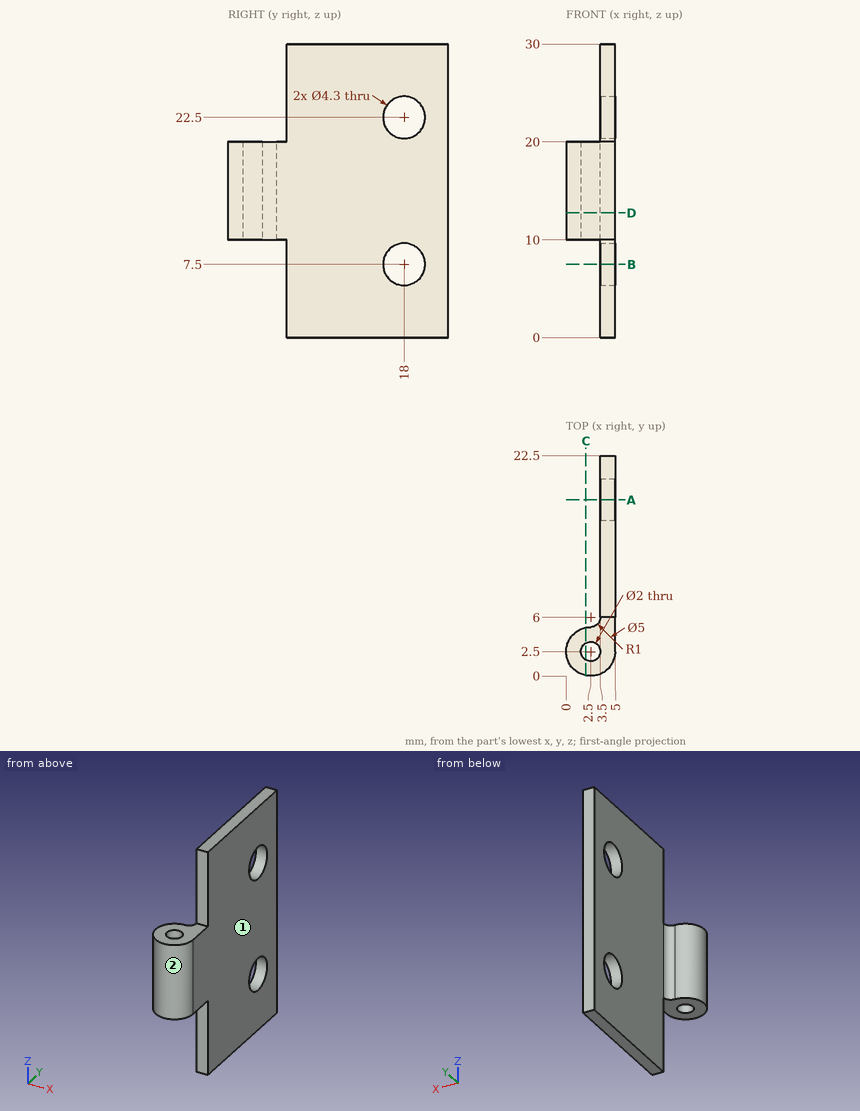
Study the drawing (mm; zero at the part's minimum x, y, z) and answer. Give positions to 0.01 mm unless a question says otherwise; leave off trailing zeros. Write each loop counter-clockwise with the first axis right and the second up, starting at its lowest first coordinate (ties: lowest second). Pieces come first, ordered by that corner, then holes. Notation, with made-up numbers: M 57.25,24 L 62.25,24 A24 ccw 62.25,52 Z; hole C 80,74 d3. An arc over 180 degrees is marked long. Put each result on its own line as item: value. Start each with the question number.
1. Consider line 1 along Z through (x, y) = (3.85, 18); line 2 along Y through (x, z) = (4.5, 22.5); line 3 along X through (y, z) = (15.75, 16). Determine where each line is inside the solid, lowest interval first.
2. For a pull along Y with two mould halves and no side action, classify the marked faces 1 and 2 as released by +Y, released by -Y, zero draft, split by the parting line, or undercut.
3. Each of these flat-tipped pins is pushed along its axis until it touches: pin 1 Ø5 at (y, z) = (18, 22.5) entering from -X; pin 2 Ø2.5 at (x, y) = (3.5, 2) entering from -Z; pin 3 Ø2.5 at (x, y) = (3.5, 1.5) entering from +Z. Where does it stop, or does it pass through?
4. The part is cut by section A-A, the plane y = 18. Give the vertices of the cut face in (x, z).
5. The part is cut by section B-B, the plane z = 7.5. Give the vertices of the cut face in (x, y), and give its area (3 significant figures).
6. The part is cut by section C-C, the plane x = 2. Give the vertices of the cut face in (y, z), and give its area (3 significant figures).
7. The part is cut by section D-D, the plane z = 12.75. Give the vertices of the cut face in (x, y), and give its area (3 significant figures).
Final values:
1. line 1: z = 0 to 5.35, 9.65 to 20.35, 24.65 to 30
1. line 2: y = 6 to 15.85, 20.15 to 22.5
1. line 3: x = 3.5 to 5
2. face 1: zero draft
2. face 2: split by the parting line
3. pin 1: stops at x = 3.5
3. pin 2: stops at z = 10
3. pin 3: stops at z = 20
4. outline: M 3.5,0 L 5,0 L 5,5.35 L 3.5,5.35 Z; M 3.5,9.65 L 5,9.65 L 5,20.35 L 3.5,20.35 Z; M 3.5,24.65 L 5,24.65 L 5,30 L 3.5,30 Z
5. outline: M 3.5,6 L 5,6 L 5,15.85 L 3.5,15.85 Z; M 3.5,20.15 L 5,20.15 L 5,22.5 L 3.5,22.5 Z
5. area: 18.3 mm²
6. outline: M 0.05,10 L 1.63,10 L 1.63,20 L 0.05,20 Z; M 3.37,10 L 4.95,10 L 4.95,20 L 3.37,20 Z
6. area: 31.7 mm²
7. outline: M 2.5,5 A2.5 ccw long 5,2.5 L 5,22.5 L 3.5,22.5 L 3.5,6 A1 cw Z; hole C 2.5,2.5 d2
7. area: 44.3 mm²
